Read the model definition and answer for the solid it produces. Units are mm, in the model's axes. Face numbers are marked on the shaded views. A direction names the side the tool comes from. Give positions to 0.01 mm unless a question says otherwise; leave off trailing zeros. Order: outer loops, then holes, each group sorted by start corner. A loop starts at its lowest first (then second) coordinate and runs counter-clockwise, first axis right, second up.
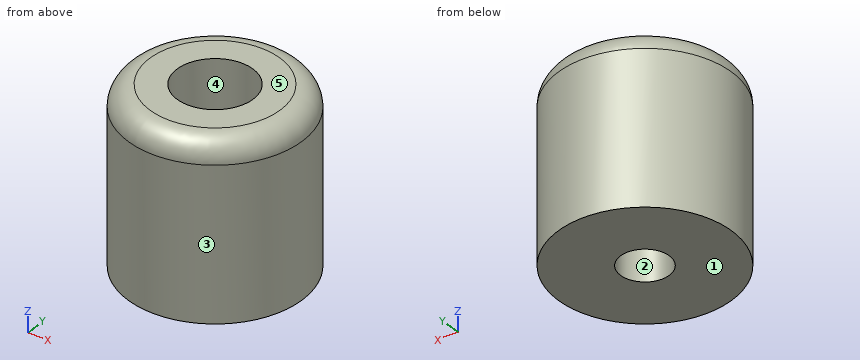
```python
from build123d import *

# Parameters (mm, degrees)
SKETCH1_R           = 12.7
SKETCH1_R_2         = 3.571875
BOSS_EXTRUDE1_DEPTH = 25.4
SKETCH2_R           = 5.55625
CUT_EXTRUDE1_DEPTH  = 12.7
FILLET1_R           = 3.175


with BuildPart() as part:
    # Sketch1 → Boss-Extrude1 (new body)
    with BuildSketch(Plane.XY):
        Circle(SKETCH1_R)
        Circle(SKETCH1_R_2, mode=Mode.SUBTRACT)
    extrude(amount=BOSS_EXTRUDE1_DEPTH)

    # Sketch2 → Cut-Extrude1 (cut)
    with BuildSketch(Plane.XY.offset(25.4)):
        Circle(SKETCH2_R)
    extrude(amount=-CUT_EXTRUDE1_DEPTH, mode=Mode.SUBTRACT)

    # Fillet1
    fillet1_edges = [part.edges().sort_by_distance(p)[0] for p in [
        (-12.7, 0, 25.4),
    ]]
    fillet(fillet1_edges, radius=FILLET1_R)


solid = part.part
```
1) Consider L1, parallel to Y at x = 0, z = 6; L2, parallel to Y at x = 0, z = 18; L3, parallel to Z at x = 9.25, y = -2.75. Determine where each line is inside the solid, lowest interval first.
Final values:
L1: y = -12.7 to -3.57, 3.57 to 12.7
L2: y = -12.7 to -5.56, 5.56 to 12.7
L3: z = 0 to 25.4
2) Given pin 1 (1 mm diameter, centred on x = 0.5, z = 22, fed in from -Y); pin 2 (4 mm diameter, centred on x = -7, z = 18.5, fed in from -Y); pin 3 (6 mm diameter, centred on y = -10, z = 16.5, fed in from +X); pin 4 (10 mm diameter, centred on y = 8, z = 3.5, fed in from -X), each flat-ended and moving along its own axis, determine where each tip first touches the part or whether it passes through.
Final values:
pin 1: stops at y = -12.7
pin 2: stops at y = -11.67
pin 3: stops at x = 10.6
pin 4: stops at x = -12.34
3) A tool of negligible diameter and unlimited length cuts with its end or side. For the marked faces 4 and 5, from which of +Z, -Z, +X, -X, +Y, -Y can it reach the whole face along a straight path? Write none if from no direction.
Final values:
face 4: +Z
face 5: +Z, +X, -X, +Y, -Y
4) The part is cut by section A-A on x = 0. Determine the outline of the cut face in (y, z) (3 decimals), and give its area (3 significant figures).
Final values:
outline: (-12.7, 0) - (-3.572, 0) - (-3.572, 12.7) - (-5.556, 12.7) - (-5.556, 25.4) - (-9.525, 25.4) arc R3.175 ccw to (-12.7, 22.225) - close; (3.572, 0) - (12.7, 0) - (12.7, 22.225) arc R3.175 ccw to (9.525, 25.4) - (5.556, 25.4) - (5.556, 12.7) - (3.572, 12.7) - close
area: 409 mm2
5) For a pull along X with two mould halves and no side action, classify the marked faces 1, 2 and 3 as released by +X, released by -X, zero draft, split by the parting line, or undercut.
Final values:
face 1: zero draft
face 2: undercut
face 3: split by the parting line
6) The part is cut by section C-C on z = 21.5. Determine the outline of the cut face in (x, y), and give its area (3 significant figures).
Final values:
outline: circle Ø25.4 at (0, 0); hole circle Ø11.11 at (0, 0)
area: 410 mm2
7) The part is cut by section D-D on z = 2.5. Determine the outline of the cut face in (x, y), and give its area (3 significant figures).
Final values:
outline: circle Ø25.4 at (0, 0); hole circle Ø7.14 at (0, 0)
area: 467 mm2
